Autodesk Fusion 360 part; units mm, degrees
sketch "Sketch1" plane through (0, 0, 0) normal (0, 0, 1) x (1, 0, 0)
  circle A0 centre (0, 0) radius 16.5
  circle A1 centre (0, 0) radius 12.5
  dimension "d1" = 33
  dimension "d2" = 25
extrude "Extrude1" add sketch "Sketch1" along normal blind 8
sketch "Sketch2" plane through (0, 0, 8) normal (0, 0, 1) x (-1, 0, 0)
  circle A0 centre (0, 0) radius 12.5
  circle A1 centre (0, 0) radius 16.5
  line L0 (-0.0363, -16.5) -> (-0.0363, -1.5) construction
  line L1 (-0.0363, -1.5) -> (16.4317, -1.5) construction
  line L2 (16.4317, -1.5) -> (-16.4317, -1.5)
  line L3 (-16.4317, -1.5) -> (-13.3757, -8.3419)
  dimension "d5" = 15
  dimension "d6" = 7.4934
extrude "Extrude2" add sketch "Sketch2" along normal blind 5 contours A0 A1 L2 picked at (14.9574, -2.302)
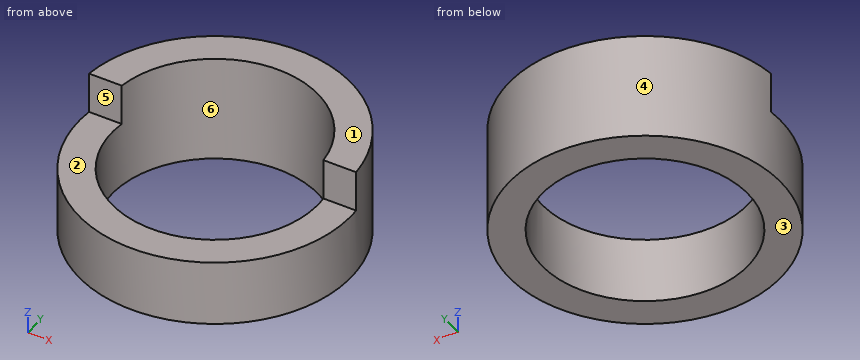
Source: CAD feature listing. Evaluate the final solid. Frame: model axes, mm. Face numbers are marked on the shaded views. A direction names the side the tool comes from. Coordinates: 2 decimals unless noted, no trailing zeros. Order: outer loops, then holes, each group sorted by start corner. A loop starts at its lowest first (then second) coordinate and runs counter-clockwise, first axis right, second up. Notation, with made-up numbers: M -14.75,0 L 0.25,0 A14 ccw 0.25,4 Z; hole C -31,11 d5. An arc over 180 degrees is marked long. Write each question's results on one line, items separated by ' | '. Start each with the question number.
Item 1: Cut plane D-D (y = -14). Return loops of the section in (x, z), and give its area (3 significant figures).
Item 2: Cut plane C-C (z = 1.75). Return loops of the section in (x, y).
Item 3: Cut plane B-B (x = 0). Return loops of the section in (y, z), and give its area (3 significant figures).
Item 4: Draft query along Y for the marked faces 3, 4, 5 and 6. Return one class per face: pulls with the +Y half, pulls with the -Y half, needs draft (parallel to the pull), parting line crosses it, or undercut.
Item 5: Set-up query: the marked faces 1 and 2. Return all of +Z, -Z, +X, -X, +Y, -Y with unobstructed straight access to the full face (end or side cutting, diameter ignored); none if empty.
Item 6: Cut plane A-A (y = 0). Return loops of the section in (x, z).
Item 7: Line query: probe 1 along Y at (x, z) = (0, 4.25); probe 2 along Y at (x, z) = (0, 9.25). Output: solid intervals per line, ascending.
Item 8: First-contact query: pin 1 Ø6 at (x, y) = (-6, -8.5) entering from +Z; pin 2 Ø5 at (x, z) = (-12.5, 4.5) entering from +Y; pin 3 Ø2 at (x, z) = (-14.5, 10) entering from -Y. Flat tips, straight axial feed; report the tip coordinate or a pass-through.
Checked values:
1) outline: M -8.73,0 L 8.73,0 L 8.73,8 L -8.73,8 Z | area: 140 mm2
2) outline: C 0,0 d33; hole C 0,0 d25
3) outline: M -16.5,0 L -12.5,0 L -12.5,8 L -16.5,8 Z; M 12.5,0 L 16.5,0 L 16.5,13 L 12.5,13 Z | area: 84.0 mm2
4) face 3: needs draft | face 4: parting line crosses it | face 5: pulls with the -Y half | face 6: undercut
5) face 1: +Z, +X, -X, +Y, -Y | face 2: +Z, +X, -X, -Y
6) outline: M -16.5,0 L -12.5,0 L -12.5,8 L -16.5,8 Z; M 12.5,0 L 16.5,0 L 16.5,8 L 12.5,8 Z
7) probe 1: y = -16.5 to -12.5, 12.5 to 16.5 | probe 2: y = 12.5 to 16.5
8) pin 1: stops at z = 8 | pin 2: stops at y = 13.12 | pin 3: stops at y = 1.5
